Verification items for the finished model (mm, model axes). Face numbers are marked on the shaded views. Give positions to 0.01 mm unless a question says otherwise; leave off trailing zeros. Order: outer loops, then holes, each group sorted by start corner. A loop starts at its lowest first (then second) coordinate and runs counter-clockwise, first axis right, second up. Notation, with made-up numbers: (62.25, -8) -> (103.25, -8) arc R18 cw to (103.25, 12) -> close; hole circle Ø6 at (-16.5, 9.5). An arc over 180 degrees is marked (long way). Return JSON: item names as keys, results as strings. Group by question number.
(1) Cross-section at B-B on y = 6.35. Enter the section's corners in (x, z).
(2) Depth check by flat-ended pin: pin 1 Ø3 at (x, y) = (0, 0) entering from +Z; pin 2 Ø5 at (x, z) = (10.5, 32) entering from +Y; pin 3 Ø4 at (x, y) = (0, 6.35) entering from -Z; pin 4 Ø3.5 at (x, y) = (0, 6.35) entering from +Z. Enter the tip coordinate at first touch or a pass-through.
(3) Cross-section at D-D on z = 3. State how many separate pieces and enclosed holes the cut face has, then the cut area to 3 significant figures.
(4) Cross-section at C-C on x = -30. Enter the section's corners in (y, z), then the cut area to 3 significant figures.
(5) Release check for a two-part mould opening along X. For the marked faces 1, 2 and 3 record: pulls with the +X half, pulls with the -X half, needs draft (parallel to the pull), parting line crosses it, or undercut.
(6) Cross-section at A-A on x = 0. Enter the section's corners in (y, z), then the cut area to 3 significant figures.
(7) Thickness scan on line 1 along Y through (x, z) = (0, 2); line 2 along Y through (x, z) = (0, 19.5); line 3 along X through (y, z) = (28, 40.5). Record the ranges inside material, lowest first.
Autodesk Inventor part; units mm, degrees
ref_plane "YZ Plane" through (0, 0, 0) normal (1, 0, 0) x (0, 1, 0)
ref_plane "XZ Plane" through (0, 0, 0) normal (0, 1, 0) x (-1, 0, 0)
ref_plane "XY Plane" through (0, 0, 0) normal (0, 0, 1) x (1, 0, 0)
sketch "Sketch1" plane through (0, 0, 0) normal (0, 0, 1) x (1, 0, 0)
  circle A0 centre (0, 0) radius 37.5
  dimension "d0" = 75
extrude "Extrusion1" add sketch "Sketch1" along normal blind 42
sketch "Sketch2" plane through (0, 0, 42) normal (0, 0, 1) x (1, 0, 0)
  circle A0 centre (0, 0) radius 10
  dimension "d3" = 20
extrude "Extrusion2" cut sketch "Sketch2" against normal blind 6
sketch "Sketch3" plane through (0, 0, 36) normal (0, 0, 1) x (1, 0, 0)
  circle A0 centre (6.35, 0) radius 1.5
  circle A1 centre (0, 6.35) radius 1.5
  circle A2 centre (-6.35, 0) radius 1.5
  circle A3 centre (0, -6.35) radius 1.5
  point P0 (0, 0)
  dimension "d6" = 3
  dimension "d7" = 6.35
  dimension "d10" = 360
extrude "Extrusion3" cut sketch "Sketch3" against normal through all
sketch "Sketch4" plane through (0, 0, 36) normal (0, 0, 1) x (1, 0, 0)
  circle A0 centre (0, 0) radius 2.5
  dimension "d14" = 5
extrude "Extrusion4" cut sketch "Sketch4" against normal through all
sketch "Sketch5" plane through (0, 0, 0) normal (0, 0, -1) x (-1, 0, 0)
  circle A0 centre (6.35, 0) radius 1.5
  circle A1 centre (6.35, 0) radius 3.5
  circle A2 centre (0, 6.35) radius 3.5
  circle A3 centre (-6.35, 0) radius 3.5
  circle A4 centre (0, -6.35) radius 3.5
  point P0 (0, 0)
  dimension "d17" = 7
  dimension "d20" = 360
extrude "Extrusion5" cut sketch "Sketch5" against normal blind 4 contours A0 | A1 | A2 | A3 | A4
sketch "Sketch6" plane through (0, 0, 0) normal (0, 0, -1) x (-1, 0, 0)
  circle A0 centre (-30, 0) radius 2.5
  circle A1 centre (-15, -25.9808) radius 2.5
  circle A2 centre (15, -25.9808) radius 2.5
  circle A3 centre (30, 0) radius 2.5
  circle A4 centre (15, 25.9808) radius 2.5
  circle A5 centre (-15, 25.9808) radius 2.5
  point P0 (0, 0)
  dimension "d24" = 5
  dimension "d25" = 30
  dimension "d28" = 360
extrude "Extrusion6" cut sketch "Sketch6" against normal through all
properties part number "HA012" material "ABS Plastic"
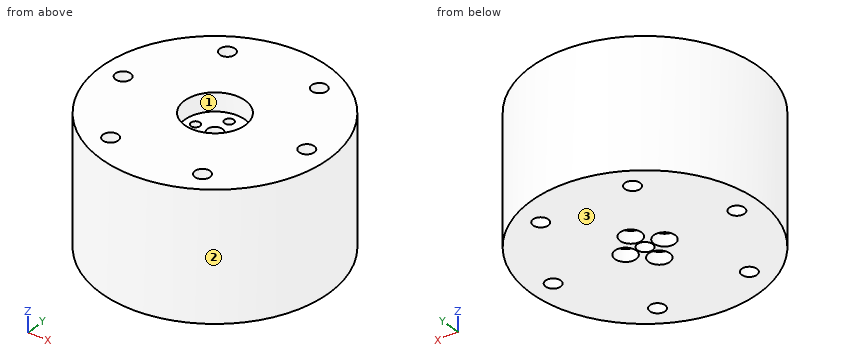
Verdict:
{
 "1": {"outline": "(-36.96, 0) -> (-3.5, 0) -> (-3.5, 4) -> (-1.5, 4) -> (-1.5, 36) -> (-7.73, 36) -> (-7.73, 42) -> (-36.96, 42) -> close; (1.5, 4) -> (3.5, 4) -> (3.5, 0) -> (36.96, 0) -> (36.96, 42) -> (7.73, 42) -> (7.73, 36) -> (1.5, 36) -> close"},
 "2": {"pin 1": "through", "pin 2": "y = 36.64", "pin 3": "z = 4", "pin 4": "z = 36"},
 "3": {"separate pieces": "1", "enclosed holes": "11", "area": "4,130 mm²"},
 "4": {"outline": "(-22.5, 0) -> (-2.5, 0) -> (-2.5, 42) -> (-22.5, 42) -> close; (2.5, 0) -> (22.5, 0) -> (22.5, 42) -> (2.5, 42) -> close", "area": "1,680 mm²"},
 "5": {"face 1": "undercut", "face 2": "parting line crosses it", "face 3": "needs draft"},
 "6": {"outline": "(-37.5, 0) -> (-9.85, 0) -> (-9.85, 4) -> (-7.85, 4) -> (-7.85, 36) -> (-10, 36) -> (-10, 42) -> (-37.5, 42) -> close; (-4.85, 4) -> (-2.85, 4) -> (-2.85, 0) -> (-2.5, 0) -> (-2.5, 36) -> (-4.85, 36) -> close; (2.5, 0) -> (2.85, 0) -> (2.85, 4) -> (4.85, 4) -> (4.85, 36) -> (2.5, 36) -> close; (7.85, 4) -> (9.85, 4) -> (9.85, 0) -> (37.5, 0) -> (37.5, 42) -> (10, 42) -> (10, 36) -> (7.85, 36) -> close", "area": "2,600 mm²"},
 "7": {"line 1": "-37.5 to -9.85, -2.85 to -2.5, 2.5 to 2.85, 9.85 to 37.5", "line 2": "-37.5 to -7.85, -4.85 to -2.5, 2.5 to 4.85, 7.85 to 37.5", "line 3": "-24.94 to -16.47, -13.53 to 13.53, 16.47 to 24.94"}
}
